Check sheet for the modelled part. Datum: model origin and axes. Units: mm. A direction names the side the tool comes from. Give positions to 0.01 mm unless a question says otherwise; leave off trailing zeros. Order: outer loops, then holes, each group sorted by start corner. A loop starts at its lowest first (then second) coordinate and runs counter-clockwise, first axis right, second up.
```python
from build123d import *

# Parameters (mm, degrees)
SKETCH1_R           = 3.302
BOSS_EXTRUDE1_DEPTH = 6.35
FILLET1_R           = 3.175
SKETCH2_R           = 1.905
CUT_EXTRUDE2_DEPTH  = 6.35
BOSS_EXTRUDE2_START = -6.35
SKETCH3_R           = 1.524
BOSS_EXTRUDE2_DEPTH = 6.35


with BuildPart() as part:
    # Sketch1 → Boss-Extrude1 (new body)
    # profile 1 of 8: a face of its own
    with BuildSketch(Plane.XY):
        with BuildLine():
            Line((141.278581179, 57.15), (154.893148654, 57.15))
            ThreePointArc((154.893148654, 57.15), (149.477461353, 70.103484559), (142.980794165, 82.55))
            Line((142.980794165, 82.55), (136.957419152, 82.55))
            Line((136.957419152, 82.55), (136.957419152, 66.846281418))
            ThreePointArc((136.957419152, 66.846281418), (139.202451266, 62.035776465), (141.278581179, 57.15))
        make_face()
    # profile 2 of 8: a face of its own
    with BuildSketch(Plane.XY):
        with BuildLine():
            Line((154.893148654, 57.15), (165.008388044, 57.15))
            ThreePointArc((165.008388044, 57.15), (159.949723048, 70.071226062), (153.881084364, 82.55))
            Line((153.881084364, 82.55), (142.980794165, 82.55))
            ThreePointArc((142.980794165, 82.55), (149.477461353, 70.103484559), (154.893148654, 57.15))
        make_face()
    # profile 3 of 8: a face of its own
    with BuildSketch(Plane.XY):
        with BuildLine():
            Line((165.008388044, 57.15), (165.532419152, 57.15))
            ThreePointArc((165.532419152, 57.15), (173.560812364, 66.556688744), (184.112113246, 60.106034483))
            ThreePointArc((184.112113246, 60.106034483), (180.006858286, 71.467031526), (175.201321699, 82.55))
            Line((175.201321699, 82.55), (153.881084364, 82.55))
            ThreePointArc((153.881084364, 82.55), (159.949723048, 70.071226062), (165.008388044, 57.15))
        make_face()
    # profile 4 of 8: a face of its own
    with BuildSketch(Plane.XY):
        with BuildLine():
            ThreePointArc((184.112113246, 60.106034483), (184.587488278, 58.629896777), (185.051028435, 57.15))
            Line((185.051028435, 57.15), (194.997737166, 57.15))
            Line((194.997737166, 57.15), (200.457419152, 57.15))
            Line((200.457419152, 57.15), (200.457419152, 82.55))
            Line((200.457419152, 82.55), (175.201321699, 82.55))
            ThreePointArc((175.201321699, 82.55), (180.006858286, 71.467031526), (184.112113246, 60.106034483))
        make_face()
        with Locations((190.932419152, 73.025)):
            Circle(SKETCH1_R, mode=Mode.SUBTRACT)
    # profile 5 of 8: a face of its own
    with BuildSketch(Plane.XY):
        with BuildLine():
            Line((165.532419152, 57.15), (175.057419152, 57.15))
            Line((175.057419152, 57.15), (185.051028435, 57.15))
            ThreePointArc((185.051028435, 57.15), (184.587488278, 58.629896777), (184.112113246, 60.106034483))
            ThreePointArc((184.112113246, 60.106034483), (173.560812364, 66.556688744), (165.532419152, 57.15))
        make_face()
    # profile 6 of 8: a face of its own
    with BuildSketch(Plane.XY):
        with BuildLine():
            Line((185.051028435, 57.15), (175.057419152, 57.15))
            ThreePointArc((175.057419152, 57.15), (179.769184167, 39.92822215), (182.790987009, 22.331089728))
            ThreePointArc((182.790987009, 22.331089728), (185.361789246, 21.512549972), (186.464004794, 19.05))
            ThreePointArc((186.464004794, 19.05), (185.604733587, 16.828225925), (183.474131965, 15.762785278))
            ThreePointArc((183.474131965, 15.762785278), (183.905882161, 9.478871593), (184.122474139, 3.183868229))
            ThreePointArc((184.122474139, 3.183868229), (190.813712192, 6.352963326), (193.213868393, 13.356896552))
            ThreePointArc((193.213868393, 13.356896552), (190.395751057, 35.488922277), (185.051028435, 57.15))
        make_face()
    # profile 7 of 8: a face of its own
    with BuildSketch(Plane.XY):
        with BuildLine():
            ThreePointArc((182.790987009, 22.331089728), (179.769184167, 39.92822215), (175.057419152, 57.15))
            Line((175.057419152, 57.15), (165.538614463, 56.806514484))
            ThreePointArc((165.538614463, 56.806514484), (165.679249432, 55.483999485), (166.002725058, 54.193965517))
            ThreePointArc((166.002725058, 54.193965517), (171.406582826, 33.37175436), (174.209225601, 12.043103448))
            ThreePointArc((174.209225601, 12.043103448), (177.364510323, 5.597834805), (184.122474139, 3.183868229))
            ThreePointArc((184.122474139, 3.183868229), (183.905882161, 9.478871593), (183.474131965, 15.762785278))
            ThreePointArc((183.474131965, 15.762785278), (179.87772057, 18.708413793), (182.790987009, 22.331089728))
        make_face()
    # profile 8 of 8: a face of its own
    with BuildSketch(Plane.XY):
        with BuildLine():
            Line((165.538614463, 56.806514484), (175.057419152, 57.15))
            Line((175.057419152, 57.15), (165.532419152, 57.15))
            ThreePointArc((165.532419152, 57.15), (165.533968105, 56.978229309), (165.538614463, 56.806514484))
        make_face()
    extrude(amount=BOSS_EXTRUDE1_DEPTH)

    # Fillet1
    fillet1_edges = [part.edges().sort_by_distance(p)[0] for p in [
        (136.957419152, 82.55, 3.175),
        (200.457419152, 82.55, 3.175),
        (200.457419152, 57.15, 3.175),
    ]]
    fillet(fillet1_edges, radius=FILLET1_R)

    # Sketch2 → Cut-Extrude2 (cut)
    with BuildSketch(Plane.XY.offset(6.35)):
        with Locations((149.657419152, 76.2)):
            Circle(SKETCH2_R)
        with Locations((152.832419152, 66.675)):
            Circle(SKETCH2_R)
    extrude(amount=-CUT_EXTRUDE2_DEPTH, mode=Mode.SUBTRACT)

    # Sketch3 → Boss-Extrude2 (add)
    with BuildSketch(Plane.XY.offset(6.35).offset(BOSS_EXTRUDE2_START)):
        with BuildLine():
            ThreePointArc((172.000332031, 30.1625), (170.759719622, 36.537771957), (169.282889622, 42.8625))
            Line((169.282889622, 42.8625), (156.561270912, 32.229125785))
            ThreePointArc((156.561270912, 32.229125785), (156.072362343, 25.392696876), (162.921852432, 25.147182454))
            Line((162.921852432, 25.147182454), (168.121534475, 30.1625))
            Line((168.121534475, 30.1625), (172.000332031, 30.1625))
        make_face()
        with Locations((159.615574597, 28.575)):
            Circle(SKETCH3_R, mode=Mode.SUBTRACT)
    extrude(amount=BOSS_EXTRUDE2_DEPTH)


solid = part.part
```
(1) Sectioned sample at B-B (y = 11). Enter the section's corners in (x, z), plus the area to 3 significant figures.
(2) Thickness scan on L1, parallel to X at y = 27.5, z = 3.5; L2, parallel to X at y = 26, z = 3.25; L3, parallel to X at y = 73, z = 1.25. Record the ranges inside material, lowest first.
(3) Sectioned sample at A-A (z = 4). Count the separate pieces of the cut face and the enclosed holes in it, plus the area to 3 significant figures.
(4) Go/stop test with flat-tipped pins: P1, Ø2, axis at x = 151, z = 0.5, coming from the -Y side; P2, Ø3, axis at x = 158.5, z = 5.5, coming from the -Y side; P3, Ø1, axis at x = 155, z = 5.5, coming from the -Y side. Record where each tip stops, or that it passes through.
(5) Release check for a two-part mould opening along Y. For faces 1 (the face through (199.55, 58.1, 3.22)), 2 (the face through (169, 82.55, 3)), 3 (the face through (158.093, 28.642, 3.131)) record: released by +Y, released by -Y, zero draft, split by the parting line, or undercut.
(6) Tool access check on faces 4 (the face through (137.863, 81.595, 3.219)), 5 (the face through (167.716, 48.635, 3.131)), 6 (the face through (175, 52, 0)), 7 (the face through (191, 57.15, 3)), 8 (the face through (165.485, 27.62, 3.131)). Record the directions out of +Z, -Z, +X, -X, +Y, -Y that give a thin tool (end or side, any length) a straight path to the whole face; none if there is none.
Values follow:
1. outline: (174.34, 0) - (193.08, 0) - (193.08, 6.35) - (174.34, 6.35) - close
1. area: 119 mm2
2. L1: x = 154.98 to 158.54, 160.7 to 165.36, 172.45 to 191.71
2. L2: x = 155.61 to 163.81, 172.68 to 191.92
2. L3: x = 136.96 to 187.63, 194.23 to 200.46
3. separate pieces: 1
3. enclosed holes: 5
3. area: 2,660 mm2
4. P1: stops at y = 57.15
4. P2: stops at y = 23.81
4. P3: stops at y = 26.18
5. face 1: released by -Y
5. face 2: released by +Y
5. face 3: undercut
6. face 4: +Z, -Z, -X, +Y
6. face 5: +Z, -Z, -X
6. face 6: -Z, +X, -X, +Y, -Y
6. face 7: +Z, -Z, +X
6. face 8: +Z, -Z, -Y
